Source: CAD feature listing. Evaluate the final solid. Frame: model axes, mm. Give positions to 0.01 mm unless a question says otherwise; leave off trailing zeros. Order: outer loops, then holes, each group sorted by start corner. A loop starts at its lowest first (then second) coordinate and runs counter-clockwise, first axis right, second up. Notation, with made-up numbers: M -30,14 L -15,14 A23 ccw -15,45 Z; hole C 44.25,66.25 d2. An arc over 180 degrees is marked long. Answer as a JSON object with one key per item and string values. Group by question number.
1. Material intervals for L1, parallel to Z at x = -12.7, y = -3.65 (3 decimals); L2, parallel to Z at x = -12, y = -6; L3, parallel to Y at x = -8.5, z = 13.5, sorted ascending. Write a range as [from, to].
2. Section query B-B (y = -2.25). Count the separate pieces of the cut face and the enclosed holes in it, plus the area to 3 significant figures.
3. Pin query (flat end, axial travel): P1, Ø5, axis at x = -25.4, z = 12.7, coming from the +Y side; P2, Ø8.5, axis at x = 38.1, z = -12.7, coming from the -Y side (3 decimals); P3, Ø10, axis at x = -12.7, z = 12.7, coming from the -Y side. Return the tip coordinate at first contact, or that it passes through.
4. Section query A-A (x = 0). Output: boundary loops of the cut face in (y, z) (3 decimals), plus the area to 3 significant figures.
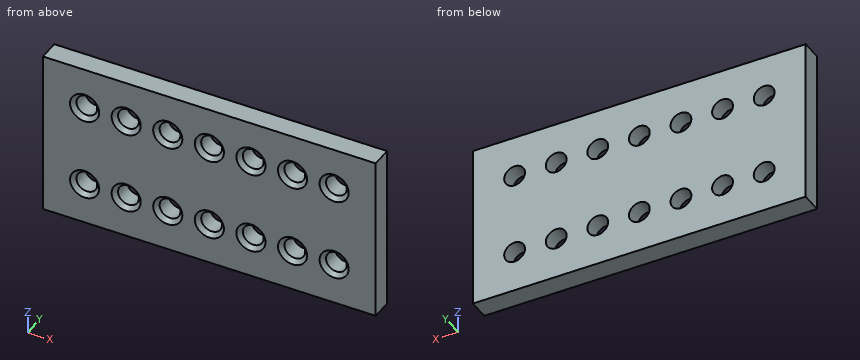
from build123d import *

# Parameters (mm, degrees)
F0_W     = 101.6
F0_H     = 50.8
F0_R     = 3.175
F1_DEPTH = 6.35
F2_SIZE  = 1.27


with BuildPart() as f1:
    # F0 (on Front) → F1 (new body)
    with BuildSketch(Plane.XZ):
        Rectangle(F0_W, F0_H)
        with Locations((-38.1, -12.7)):
            Circle(F0_R, mode=Mode.SUBTRACT)
        with Locations((-25.4, -12.7)):
            Circle(F0_R, mode=Mode.SUBTRACT)
        with Locations((-12.7, -12.7)):
            Circle(F0_R, mode=Mode.SUBTRACT)
        with Locations((0, -12.7)):
            Circle(F0_R, mode=Mode.SUBTRACT)
        with Locations((12.7, -12.7)):
            Circle(F0_R, mode=Mode.SUBTRACT)
        with Locations((25.4, -12.7)):
            Circle(F0_R, mode=Mode.SUBTRACT)
        with Locations((38.1, -12.7)):
            Circle(F0_R, mode=Mode.SUBTRACT)
        with Locations((-38.1, 12.7)):
            Circle(F0_R, mode=Mode.SUBTRACT)
        with Locations((-25.4, 12.7)):
            Circle(F0_R, mode=Mode.SUBTRACT)
        with Locations((-12.7, 12.7)):
            Circle(F0_R, mode=Mode.SUBTRACT)
        with Locations((0, 12.7)):
            Circle(F0_R, mode=Mode.SUBTRACT)
        with Locations((12.7, 12.7)):
            Circle(F0_R, mode=Mode.SUBTRACT)
        with Locations((25.4, 12.7)):
            Circle(F0_R, mode=Mode.SUBTRACT)
        with Locations((38.1, 12.7)):
            Circle(F0_R, mode=Mode.SUBTRACT)
    extrude(amount=F1_DEPTH)

    # F2
    f2_edges = [f1.edges().sort_by_distance(p)[0] for p in [
        (-41.275, -6.35, 12.7),
        (-28.575, -6.35, 12.7),
        (-15.875, -6.35, 12.7),
        (-3.175, -6.35, 12.7),
        (9.525, -6.35, 12.7),
        (22.225, -6.35, 12.7),
        (34.925, -6.35, 12.7),
        (34.925, -6.35, -12.7),
        (22.225, -6.35, -12.7),
        (9.525, -6.35, -12.7),
        (-3.175, -6.35, -12.7),
        (-15.875, -6.35, -12.7),
        (-41.275, -6.35, -12.7),
        (-28.575, -6.35, -12.7),
    ]]
    chamfer(f2_edges, length=F2_SIZE)


solid = f1.part
Answer sheet:
{
 "1": {"L1": "[-25.4, -15.875], [-9.525, 9.525], [15.875, 25.4]", "L2": "[-25.4, -16.73], [-8.67, 8.67], [16.73, 25.4]", "L3": "[-6.18, 0]"},
 "2": {"separate pieces": "1", "enclosed holes": "14", "area": "4,720 mm^2"},
 "3": {"P1": "through", "P2": "y = -6.155", "P3": "y = -6.35"},
 "4": {"outline": "M -6.35,-25.4 L 0,-25.4 L 0,-15.875 L -5.08,-15.875 L -6.35,-17.145 Z; M -6.35,-8.255 L -5.08,-9.525 L 0,-9.525 L 0,9.525 L -5.08,9.525 L -6.35,8.255 Z; M -6.35,17.145 L -5.08,15.875 L 0,15.875 L 0,25.4 L -6.35,25.4 Z", "area": "239 mm^2"}
}
